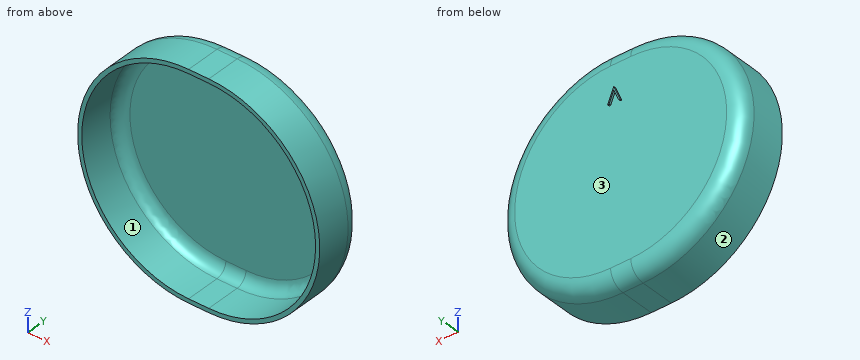
```python
from build123d import *

# Parameters (mm, degrees)
SKETCH3_W                = 12.333298302
SKETCH3_H                = 1
BOSS_EXTRUDE1_DEPTH      = 4
BOSS_EXTRUDE1_DEPTH_BACK = 1
BOSS_EXTRUDE2_DEPTH      = 0.5


with BuildPart() as part:
    # Sweep1: sweep along a path in Sketch1
    with BuildLine(Plane(origin=(0, -28.156757597, 0), x_dir=(1, 0, 0), z_dir=(0, 1, 0))) as sweep1_path:
        Line((1.032552653, 27.955195416), (-3.837557561, 27.953997551))
        ThreePointArc((-3.837557561, 27.953997551), (-29.664515825, 2.114331239), (-3.824849512, -23.712627024))
        Line((-3.824849512, -23.712627024), (1.045260702, -23.71142916))
        ThreePointArc((1.045260702, -23.71142916), (26.872218965, 2.128237152), (1.032552653, 27.955195416))
    # Sketch2 → Sweep1 (sweep)
    with BuildSketch(Plane(origin=(0, 0, 0), x_dir=(0, 0, -1), z_dir=(1, 0, 0))):
        with BuildLine():
            Line((27.954596483, -28.156757597), (27.954596483, -19.795322572))
            ThreePointArc((27.954596483, -19.795322572), (27.181778695, -17.929575385), (25.316031508, -17.156757597))
            Line((25.316031508, -17.156757597), (3.413395706, -17.156757597))
            Line((3.413395706, -17.156757597), (3.413395706, -16.156757597))
            Line((3.413395706, -16.156757597), (25.316031508, -16.156757597))
            ThreePointArc((25.316031508, -16.156757597), (27.888885476, -17.222468604), (28.954596483, -19.795322572))
            Line((28.954596483, -19.795322572), (28.954596483, -28.156757597))
            Line((28.954596483, -28.156757597), (27.954596483, -28.156757597))
        make_face()
    sweep(path=sweep1_path.line)

    # Sketch3 → Boss-Extrude1 (add, two sides)
    with BuildSketch(Plane(origin=(-0.000839567, 0, -3.4133955), x_dir=(0.99999997, 0, -0.000245962), z_dir=(0.000245962, 0, 0.99999997))) as boss_extrude1_sk:
        with Locations((-1.731029698, -16.656757597)):
            Rectangle(SKETCH3_W, SKETCH3_H)
    extrude(amount=BOSS_EXTRUDE1_DEPTH)
    extrude(boss_extrude1_sk.sketch, amount=-BOSS_EXTRUDE1_DEPTH_BACK)

    # Sketch4 → Boss-Extrude2 (add)
    with BuildSketch(Plane(origin=(0, -16.156757597, 0), x_dir=(1, 0, 0), z_dir=(0, 1, 0))):
        Polygon((-1.641529651, -12.033441663), (-1.30499119, -12.033441663), (-0.138324523, -14.791654805), (1.028342144, -12.033441663), (1.364880605, -12.033441663), (-0.115888626, -15.533441663), (-0.160760421, -15.533441663), align=None)
    extrude(amount=BOSS_EXTRUDE2_DEPTH)


solid = part.part
```
Design review of the part built by this model. Coordinates are the model's own, in mm. Face numbers are marked on the shaded views. Give positions to 0.01 mm unless a question says otherwise; leave off trailing zeros. Write each loop counter-clockwise with the first axis right and the second up, starting at its lowest first coordinate (ties: lowest second). Pieces come first, ordered by that corner, then holes. Notation, with made-up numbers: (51.5, -24.75) - (110.5, -24.75) arc R10 cw to (110.5, -8.75) - close; hole circle Ø2 at (58, 82). An arc over 180 degrees is marked (long way). Return JSON: item names as keys, results as strings. Group by question number.
(1) Mouldability with a two-part tool opening along Z and no side actions: class the marked faces 1, 2 and 3 as +Z half, -Z half, draft (parallel to the pull), parting line (faces both ways), or undercut.
(2) To check wall thickness, follow probe 1 along Z at (x, y) = (-3, -26.75); probe 2 along Y at (x, z) = (-17.5, 1.5); probe 3 along X at (y, z) = (-23.5, 4). State the ranges of each line that lie inside material, in increasing order.
(3) Insertion check: pin 1 (1.5 mm diameter, centred on x = 5.5, z = 14.5, fed in from -Y); pin 2 (5 mm diameter, centred on x = 4, y = -23.5, fed in from -Z); pin 3 (1 mm diameter, centred on y = -25, z = -14, fed in from -X). Each pin has a flat end and moves straight along its axis. Give the tip position at first contact, or say it passes through.
(4) We need section A-A, the plane y = -25.75. Give the boundary of the cut face in (x, z), then the cut area to 3 significant figures.
Reported:
{
 "1": {"face 1": "undercut", "face 2": "parting line", "face 3": "draft"},
 "2": {"probe 1": "z = -28.95 to -27.95, 23.71 to 24.71", "probe 2": "y = -17.16 to -16.16", "probe 3": "x = -29.96 to -28.93, 26.14 to 27.16"},
 "3": {"pin 1": "stops at y = -17.16", "pin 2": "stops at z = -28.95", "pin 3": "stops at x = -28.13"},
 "4": {"outline": "(-3.84, -28.95) - (1.03, -28.95) arc R26.83 ccw to (1.05, 24.71) - (-3.82, 24.71) arc R26.83 ccw to start; hole (-3.84, -27.95) - (1.03, -27.95) arc R25.83 ccw to (1.05, 23.71) - (-3.82, 23.71) arc R25.83 ccw to start", "area": "175 mm2"}
}
